Source: CAD feature listing. Evaluate the final solid. Frame: model axes, mm. Give positions to 0.01 mm unless a question says otherwise; leave off trailing zeros. Loops run counter-clockwise (first coordinate to the right, second up) from the corner with the lowest first, then second, coordinate; pieces in that order, holes last. Notation, with made-up numbers: M 7.25,17 L 32.25,17 A23 cw 32.25,55 Z; hole C 46.5,80.5 d3. An arc over 180 degrees is marked long. Write item = value, one per line.
from build123d import *

# Parameters (mm, degrees)
ESBO_O1_R                = 1.75
RESSALTO_EXTRUS_O1_DEPTH = 3


with BuildPart() as part:
    # Esboço1 → Ressalto-extrusão1 (new body)
    with BuildSketch(Plane.XY):
        Polygon((2.25, 0), (-6.25, 0), (-6.25, 2), (-6.25, 3), (-14.25, 3), (-14.25, 2), (-14.25, -42), (-14.25, -43), (-6.25, -43), (-6.25, -42), (-6.25, -40), (2.25, -40), (2.25, -36), (1, -36), (1, -33.5), (2.25, -33.5), (2.25, -31), (5.25, -31), (5.25, -33.5), (6.5, -33.5), (6.5, -36), (5.25, -36), (5.25, -40), (13.75, -40), (13.75, -42), (13.75, -43), (21.75, -43), (21.75, -42), (21.75, 2), (21.75, 3), (13.75, 3), (13.75, 2), (13.75, 0), (5.25, 0), (5.25, -4), (6.5, -4), (6.5, -6.5), (5.25, -6.5), (5.25, -9), (2.25, -9), (2.25, -6.5), (1, -6.5), (1, -4), (2.25, -4), align=None)
        with Locations((19, -5.05)):
            Circle(ESBO_O1_R, mode=Mode.SUBTRACT)
        with Locations((-11.495010855, -5.05)):
            Circle(ESBO_O1_R, mode=Mode.SUBTRACT)
        with Locations((19, -34.95)):
            Circle(ESBO_O1_R, mode=Mode.SUBTRACT)
        with Locations((-11.5, -34.95)):
            Circle(ESBO_O1_R, mode=Mode.SUBTRACT)
        Polygon((-9.95, -8.8), (-9.95, -31.2), (-9.95, -31.7), (-6.95, -31.7), (-3.95, -31.7), (-3.95, -31.2), (-3.95, -8.8), (-3.95, -8.3), (-6.95, -8.3), (-9.95, -8.3), align=None, mode=Mode.SUBTRACT)
    extrude(amount=RESSALTO_EXTRUS_O1_DEPTH)


solid = part.part
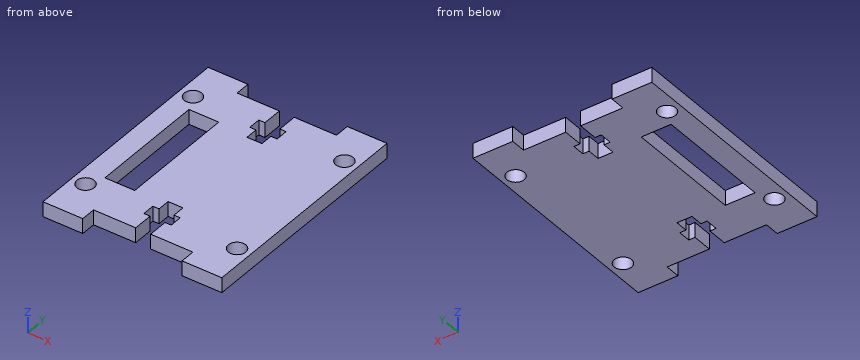
1. Material intervals for probe 1 along Y at (x, z) = (6, 2.85); probe 2 along X at (y, z) = (-4.5, 1.5); probe 3 along X at (y, z) = (-37.5, 0.85), sorted ascending. Write a range as from..to.
Derived:
probe_1 = -40..-36, -33.5..-6.5, -4..0
probe_2 = -14.25..-13.16, -9.83..1, 6.5..17.34, 20.66..21.75
probe_3 = -14.25..2.25, 5.25..21.75
2. Cut plane A-A, the plane y = -11. Return the cut outline in (x, z), then the cut area to 3 significant figures.
Derived:
outline = M -14.25,0 L -9.95,0 L -9.95,3 L -14.25,3 Z; M -3.95,0 L 21.75,0 L 21.75,3 L -3.95,3 Z
area = 90.0 mm²
3. First-contact query: pin 1 Ø1.4 at (x, z) = (1.5, 1) entering from +Y; pin 2 Ø1 at (x, z) = (2, 1.5) entering from -Y. Flat tips, straight axial feed; report the tip coordinate or a pass-through.
Derived:
pin_1 = 0
pin_2 = -40
4. Cut plane D-D, the plane z = 2.4. Count the separate pieces of the cut face and the enclosed holes in it, then the cut area to 3 significant figures.
Derived:
separate_pieces = 1
enclosed_holes = 5
area = 1,290 mm²
5. Cut plane C-C, the plane y = -34.95. Return the cut outline in (x, z).
Derived:
outline = M -14.25,0 L -13.25,0 L -13.25,3 L -14.25,3 Z; M -9.75,0 L 1,0 L 1,3 L -9.75,3 Z; M 6.5,0 L 17.25,0 L 17.25,3 L 6.5,3 Z; M 20.75,0 L 21.75,0 L 21.75,3 L 20.75,3 Z
6. Cut plane B-B, the plane x = -11.5. Return the cut outline in (y, z).
Derived:
outline = M -43,0 L -36.7,0 L -36.7,3 L -43,3 Z; M -33.2,0 L -6.8,0 L -6.8,3 L -33.2,3 Z; M -3.3,0 L 3,0 L 3,3 L -3.3,3 Z
